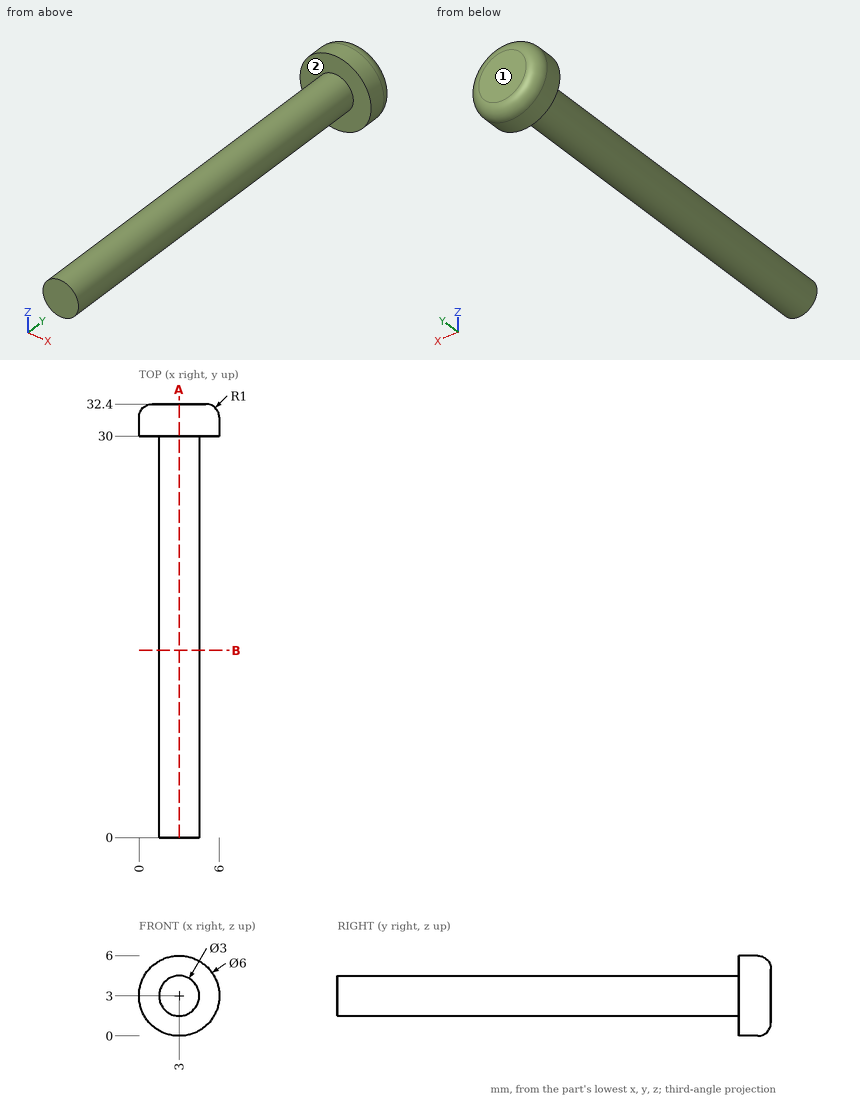
Geometry: see drawing. Coordinates: mm, zero at the bounding-box minimum. A direction names the side the tool comes from. Give positions to 0.01 mm unless a question says otherwise; leave off trailing zeros. Loops run counter-clockwise (first coordinate to the right, second up) from the corner with the lowest first, then second, coordinate; pieces in that order, holes last. Notation, with made-up numbers: (69, 27) - (119, 27) arc R25 ccw to (119, 39) - close; hole circle Ø10 at (24.25, -17.75). An arc over 180 degrees is marked (long way). Use CSV: the item, a comma, the result in double quotes. Start each with the question number.
Item 1: Line query: line 1 (Y direction, x = 1.4, z = 3.25); line 2 (Z direction, x = 1.7, y = 16); line 3 (Z direction, x = 3.4, y = 21). Output: solid intervals per line, ascending.
Item 2: Section B-B on y = 14. Return loops of the section in (x, z), then the cut area to 3 significant figures.
Item 3: Reachability of the marked faces 1 and 2 from +Z, -Z, +X, -X, +Y, -Y: full face, straight path, thin tool, end or side. Return the list, or none.
Item 4: Contact query for a flat-ended pin moving along its axis: P1, Ø1.5, axis at y = 7.5, z = 0.5, coming from the +X side. Output: stop coordinate, or through.
Item 5: Section A-A on x = 3. Return loops of the section in (y, z), then the cut area to 3 significant figures.
Ans:
1,line 1,"y = 30 to 32.4"
1,line 2,"z = 2.25 to 3.75"
1,line 3,"z = 1.55 to 4.45"
2,outline,"circle Ø3 at (3, 3)"
2,area,"7.07 mm2"
3,face 1,"+Z, -Z, +X, -X, +Y"
3,face 2,"-Y"
4,P1,"passes through"
5,outline,"(0, 1.5) - (30, 1.5) - (30, 0) - (31.4, 0) arc R1 ccw to (32.4, 1) - (32.4, 5) arc R1 ccw to (31.4, 6) - (30, 6) - (30, 4.5) - (0, 4.5) - close"
5,area,"104 mm2"
